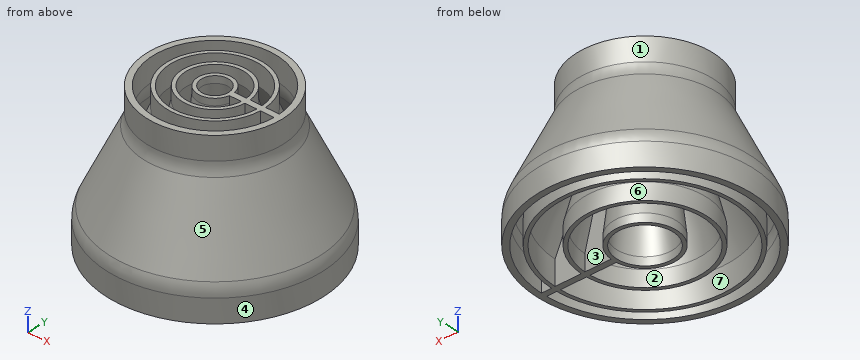
from build123d import *

# Parameters (mm, degrees)
F2_T          = -5
F6_DEPTH      = 2.5
F6_DEPTH_BACK = 2.5


with BuildPart() as f1:
    # F0 (on Front) → F1 (revolve)
    with BuildSketch(Plane.XZ):
        with BuildLine():
            Line((0, 120), (0, 0))
            Line((0, 0), (90, 0))
            Line((90, 0), (90, 19.402553))
            ThreePointArc((90, 19.402553), (89.395989, 24.864763), (87.613141, 30.063034))
            Line((87.613141, 30.063034), (59.386859, 89.936966))
            ThreePointArc((59.386859, 89.936966), (57.604011, 95.135237), (57, 100.597447))
            Line((57, 100.597447), (57, 120))
            Line((57, 120), (0, 120))
        make_face()
    revolve(axis=Axis((0, 0, 60), (0, 0, -1)))

    # F2
    f2_openings = [f1.faces().sort_by_distance(p)[0] for p in [
        (0, 0, 120),
        (0, 0, 0),
    ]]
    offset(amount=F2_T, openings=f2_openings)



with BuildPart() as f4:
    # F3 (on Front) → F4 (revolve)
    with BuildSketch(Plane.XZ):
        Polygon((11.5, 114.214671), (23.5, 6.86087), (23.5, 0), (26.5, 0), (26.5, 7.028019), (14.5, 114.38182), (14.5, 120), (11.5, 120), align=None)
        Polygon((37.5, 102.580184), (73.5, 20.51878), (73.5, 0), (76.5, 0), (76.5, 21.147887), (40.5, 103.20929), (40.5, 120), (37.5, 120), align=None)
        Polygon((24.5, 108.40939), (48.5, 13.701787), (48.5, 0), (51.5, 0), (51.5, 14.07599), (27.5, 108.783593), (27.5, 120), (24.5, 120), align=None)
    revolve(axis=Axis((0, 0, 60), (0, 0, 1)))


with BuildPart() as f1_1:
    add(f1.part)

    add(f4.part)  # F6 merges F4
    # F5 (on Front) → F6 (join, two sides)
    with BuildSketch(Plane.XZ) as f6_sk:
        Polygon((25.17798, 13.286571), (25.17798, 0), (88, 0), (88, 26.186641), (54.097552, 94.328962), (54.097552, 120), (12, 120), (12, 113.708496), align=None)
    extrude(amount=F6_DEPTH)
    extrude(f6_sk.sketch, amount=-F6_DEPTH_BACK)


solid = f1_1.part
Verification items for the finished model (mm, model axes). Face numbers are marked on the shaded views. A direction names the side the tool comes from. Give positions to 0.01 mm unless a question says otherwise; leave off trailing zeros. Write each loop counter-clockwise with the first axis right and the second up, starting at its lowest first coordinate (ties: lowest second). Pieces come first, ordered by that corner, then holes. Notation, with made-up numbers: M -13,88.25 L 11,88.25 A12 cw 11,108.25 Z; hole C -10,-22 d4. An arc over 180 degrees is marked long. Put each result on its own line as item: value. Start each with the question number.
1. Go/stop test with flat-tipped pins: pin 1 Ø3 at (y, z) = (-40.5, 51) entering from +X; pin 2 Ø8 at (x, z) = (14.5, 66) entering from -Y; pin 3 Ø1.5 at (y, z) = (18, 83) entering from -X; pin 4 Ø8 at (x, y) = (13, 50.5) entering from -Z. Record where each tip stops, or that it passes through.
2. Scan lines: line 1 along X through (y, z) = (0, 10); line 2 along X through (y, z) = (-31, 69); line 3 along Y through (x, z) = (-35, 11). Record each from-to range of solid material in increasing order. Write a range as [from, to].
3. Section check A-A (z = 47). Record the cut outline in (x, y).
4. Draft check along X on the marked faces 5, 6 and 7. Enter one of: +X half, -X half, draft (parallel to the pull), parting line (faces both ways), or undercut.
5. Section check B-B (x = 0). Give the number of separate pieces and of enclosed holes in the cut face, and give its area (3 significant figures).
6. Set-up check for the marked faces 1, 2, 3 and 4: record each of +Z, -Z, +X, -X, +Y, -Y from which the full face is reachable in a straight line by a thin tool's end or side.
Answer list:
1. pin 1: x = 67.58
1. pin 2: y = -71.24
1. pin 3: x = -60.45
1. pin 4: z = 0
2. line 1: [-90, -85], [-76.5, -73.5], [-51.5, -48.5], [-26.17, -23.15], [23.15, 90]
2. line 2: [-61.93, -55.68], [-46.04, -42.04], [-21.25, -15.11], [15.11, 21.25], [42.04, 46.04], [55.68, 61.93]
2. line 3: [-82.92, -77.46], [-68.02, -64.63], [-37.78, -33.57], [33.57, 37.78], [64.63, 68.02], [77.46, 82.92]
3. outline: C 0,0 d159.26; hole C 0,0 d38.03; hole M 21.89,-2.5 A22.03 cw long 21.89,2.5 L 39.98,2.5 A40.06 ccw long 39.98,-2.5 Z; hole M 43.08,-2.5 A43.16 cw long 43.08,2.5 L 61.83,2.5 A61.88 ccw long 61.83,-2.5 Z; hole M 65.11,-2.5 A65.16 cw long 65.11,2.5 L 74.06,2.5 A74.1 ccw long 74.06,-2.5 Z
4. face 5: parting line
4. face 6: undercut
4. face 7: undercut
5. separate pieces: 8
5. enclosed holes: 0
5. area: 3,500 mm2
6. face 1: +Z
6. face 2: -Z
6. face 3: none
6. face 4: +Z, -Z
